from build123d import *

# Parameters (mm, degrees)
SKETCH1_R                                         = 7.9375
BOSS_EXTRUDE1_DEPTH                               = 1.5875
CSK_FOR_6_FLAT_HEAD_MACHINE_SCREW_100_D           = 3.7973
CSK_FOR_6_FLAT_HEAD_MACHINE_SCREW_100_CSINK_D     = 7.0866
CSK_FOR_6_FLAT_HEAD_MACHINE_SCREW_100_CSINK_ANGLE = 100
FILLET1_R                                         = 0.254


with BuildPart() as part:
    # Sketch1 → Boss-Extrude1 (new, symmetric)
    with BuildSketch(Plane(origin=(0, 0, 0), x_dir=(1, 0, 0), z_dir=(0, 1, 0))):
        with Locations(Location((0, 0, 0), (0, 0, 270))):
            Circle(SKETCH1_R)
    extrude(amount=BOSS_EXTRUDE1_DEPTH, both=True)

    # CSK for #6 Flat Head Machine Screw (100)1 (through all)
    with Locations(Plane(origin=(0, 1.5875, 0), x_dir=(1, 0, 0), z_dir=(0, 1, 0))):
        with Locations((0, 0)):
            CounterSinkHole(CSK_FOR_6_FLAT_HEAD_MACHINE_SCREW_100_D / 2, CSK_FOR_6_FLAT_HEAD_MACHINE_SCREW_100_CSINK_D / 2, counter_sink_angle=CSK_FOR_6_FLAT_HEAD_MACHINE_SCREW_100_CSINK_ANGLE)

    # Fillet1
    fillet1_edges = [part.edges().sort_by_distance(p)[0] for p in [
        (0, -1.5875, -7.9375),
        (0, 1.5875, -7.9375),
        (3.5433, 1.5875, 0),
        (1.89865, -1.5875, 0),
        (1.89865, 0.207474792, 0),
    ]]
    fillet(fillet1_edges, radius=FILLET1_R)


solid = part.part
For this review, take the finished solid that the model builds, in its own axes (mm). Give positions to 0.01 mm unless a question says otherwise; leave off trailing zeros. Loops run counter-clockwise (first coordinate to the right, second up) from the corner with the lowest first, then second, coordinate; pieces in that order, holes last.
Item 1: Draft analysis for pull direction Z (two halves, no side actions). For faces 1 (the flat face through (-2, 1.588, -4)), 2 (the cylindrical face through (-7.75, 0.02, -1.72)), 3 (the cylindrical face through (-1.8, -0.6, -0.6)), state which applies: +Z half, -Z half, draft (parallel to the pull), parting line (faces both ways), or undercut.
Item 2: Insertion check: pin 1 (4.5 mm diameter, centred on x = 0, z = 0, fed in from -Y); pin 2 (1.5 mm diameter, centred on x = 1, y = 0.5, fed in from +Z). Each pin has a flat end and moves straight along its axis. Give the tip position at first contact, or say it passes through.
Item 3: For line 1 along X through (y, z) = (-0.85, 0); line 2 along Z through (x, y) = (-1.75, 0.7); line 3 along X through (y, z) = (0.9, -1), list the stretches that pass through material, from the lowest coordinate up.
Item 4: Take a section at A-A, the plane y = 0.65. State the section outline as (x, z) points (1 decimal), and give its area (3 significant figures).
Calculated:
1. face 1: draft
1. face 2: parting line
1. face 3: undercut
2. pin 1: stops at y = -1.59
2. pin 2: stops at z = 7.93
3. line 1: x = -7.94 to -1.9, 1.9 to 7.94
3. line 2: z = -7.74 to -1.77, 1.77 to 7.74
3. line 3: x = -7.87 to -2.53, 2.53 to 7.87
4. outline: circle Ø15.9 at (0, 0); hole circle Ø4.9 at (0, 0)
4. area: 179 mm2
